from build123d import *

# Parameters (mm, degrees)
F0_R      = 31.75
F1_DEPTH  = 25.4
F2_T      = -2.54
F3_W      = 15.6957409345
F3_H      = 22.0123222098
F3_W_2    = 15.504329931
F3_H_2    = 21.820908878
F4_DEPTH  = 58.166
F6_W      = 3.6368169822
F6_H      = 23.3522010967
F7_DEPTH  = 5.334
F8_W      = 8.804930374
F8_H      = 30.4344259202
F8_W_2    = 3.6368169822
F8_H_2    = 23.3522010967
F9_DEPTH  = 1.524
F10_R     = 6.35
F11_DEPTH = 22.86


with BuildPart() as f1:
    # F0 (on Right) → F1 (new body)
    with BuildSketch(Plane.YZ):
        Circle(F0_R)
    extrude(amount=F1_DEPTH)

    # F2
    f2_openings = [f1.faces().sort_by_distance(p)[0] for p in [
        (25.4, 0, 0),
    ]]
    offset(amount=F2_T, openings=f2_openings)

    # F3 (on Front) → F4 (cut, symmetric)
    with BuildSketch(Plane.XZ):
        with Locations((11.9632177521, 15.5043308623)):
            Rectangle(F3_W, F3_H)
        with Locations((11.8675122503, -16.9399164151)):
            Rectangle(F3_W_2, F3_H_2)
    extrude(amount=F4_DEPTH, both=True, mode=Mode.SUBTRACT)

    # F6 (on offset) → F7 (join)
    with BuildSketch(Plane.XY.offset(-29.21)):
        with Locations((9.5705741551, 0.0957059674)):
            Rectangle(F6_W, F6_H)
    extrude(amount=-F7_DEPTH)

    # F8 (on face) → F9 (join)
    with BuildSketch(Plane(origin=(0, 0, -34.544), x_dir=(1, 0, 0), z_dir=(0, 0, -1))):
        with Locations((9.4748688862, 0.5742348731)):
            Rectangle(F8_W, F8_H)
        with Locations((9.5705741551, -0.0957059674)):
            Rectangle(F8_W_2, F8_H_2, mode=Mode.SUBTRACT)
        with Locations((9.5705741551, -0.0957059674)):
            Rectangle(F8_W_2, F8_H_2)
    extrude(amount=F9_DEPTH)

    # F10 (on face) → F11 (join)
    with BuildSketch(Plane.YZ.offset(2.54)):
        Circle(F10_R)
    extrude(amount=F11_DEPTH)


solid = f1.part
Verification items for the finished model (mm, model axes). A direction names the side the tool comes from. Give positions to 0.01 mm unless a question says otherwise; leave off trailing zeros. Order: outer loops, then holes, each group sorted by start corner. A loop starts at its lowest first (then second) coordinate and runs counter-clockwise, first axis right, second up. Notation, with made-up numbers: M 76.25,25.25 L 105.25,25.25 A23 ccw 105.25,51.25 Z; hole C -32,-27.5 d3. An arc over 180 degrees is marked long. Answer as a JSON object with one key per item and string values. Group by question number.
1) Depth check by flat-ended pin: pin 1 Ø3 at (y, z) = (-7.5, -11.5) entering from +X; pin 2 Ø1.2 at (y, z) = (1, -35.5) entering from -X; pin 3 Ø2 at (x, y) = (14, -30) entering from +Z. Enter the tip coordinate at first touch or a pass-through.
2) Scan lines: line 1 along Z through (x, y) = (20, 0); line 2 along Z through (x, y) = (9.75, 0); line 3 along Y through (x, z) = (14.5, 3). Record each from-to range of solid material in increasing order. Write a range as [from, to].
3) Cross-section at B-B (y = 0). Enter the section's corners in (x, z), then the cut area to 3 significant figures.
4) Cross-section at D-D (z = 19.5). Enter the section's corners in (x, y).
5) Access from +Z, -Z, +X, -X, +Y, -Y to the whole of each face (thin tool, end or side, straight path). Record for faces 4 (the face through (10, 11.772, -32)), 5 (the face through (5.072, 0, -35)), 6 (the face through (13.877, 0, -35)), 7 (the face through (12, -30, -6.029)), 8 (the face through (12, -30, 4.498)).
6) Cross-section at A-A (z = -14). Enter the section's corners in (x, y).
7) Mould release check, pull along X, two halves, no side actions. Record for faces 1 (the face through (10, -11.58, -32)), 2 (the face through (25.4, 14, -26)), 3 (the face through (12, 30, -6.029)): released by +X, released by -X, zero draft, split by the parting line, or undercut.
8) Cross-section at C-C (z = 0). Enter the section's corners in (x, y), then the cut area to 3 significant figures.
Result sheet:
{
 "1": {"pin 1": "stops at x = 2.54", "pin 2": "stops at x = 5.07", "pin 3": "stops at z = 4.5"},
 "2": {"line 1": "z = [-31.75, -29.21], [-6.35, 6.35], [29.21, 31.75]", "line 2": "z = [-36.07, -29.21], [-6.35, 6.35], [29.21, 31.75]", "line 3": "y = [-31.61, -29.06], [-5.6, 5.6], [29.06, 31.61]"},
 "3": {"outline": "M 0,-31.75 L 7.75,-31.75 L 7.75,-34.54 L 5.07,-34.54 L 5.07,-36.07 L 13.88,-36.07 L 13.88,-34.54 L 11.39,-34.54 L 11.39,-31.75 L 25.4,-31.75 L 25.4,-29.21 L 2.54,-29.21 L 2.54,-6.35 L 25.4,-6.35 L 25.4,6.35 L 2.54,6.35 L 2.54,29.21 L 25.4,29.21 L 25.4,31.75 L 0,31.75 Z", "area": "591 mm2"},
 "4": {"outline": "M 0,-25.06 L 4.12,-25.06 L 4.12,-21.75 L 2.54,-21.75 L 2.54,21.75 L 4.12,21.75 L 4.12,25.06 L 0,25.06 Z; M 19.81,-25.06 L 25.4,-25.06 L 25.4,-21.75 L 19.81,-21.75 Z; M 19.81,21.75 L 25.4,21.75 L 25.4,25.06 L 19.81,25.06 Z"},
 "5": {"face 4": "+X, -X, +Y", "face 5": "-Z, -X, +Y, -Y", "face 6": "-Z, +X, +Y, -Y", "face 7": "-Z, -Y", "face 8": "+Z, -Y"},
 "6": {"outline": "M 0,-28.5 L 4.12,-28.5 L 4.12,-25.64 L 2.54,-25.64 L 2.54,25.64 L 4.12,25.64 L 4.12,28.5 L 0,28.5 Z; M 19.62,-28.5 L 25.4,-28.5 L 25.4,-25.64 L 19.62,-25.64 Z; M 19.62,25.64 L 25.4,25.64 L 25.4,28.5 L 19.62,28.5 Z"},
 "7": {"face 1": "zero draft", "face 2": "released by +X", "face 3": "undercut"},
 "8": {"outline": "M 0,-31.75 L 25.4,-31.75 L 25.4,-29.21 L 2.54,-29.21 L 2.54,-6.35 L 25.4,-6.35 L 25.4,6.35 L 2.54,6.35 L 2.54,29.21 L 25.4,29.21 L 25.4,31.75 L 0,31.75 Z", "area": "568 mm2"}
}
